Verification items for the finished model (mm, model axes). A direction names the side the tool comes from. Coordinates: 2 decimals unless noted, no trailing zeros. Write each loop counter-clockwise with the first axis right and the second up, starting at its lowest first coordinate (ties: lowest second). Pieces come first, ordered by that corner, then holes. Notation, with made-up numbers: (-33, 81) -> (-14, 81) arc R14 ccw to (-14, 90) -> close; hole circle Ø10 at (-3, 79). An arc over 180 degrees is marked (long way). Answer in a Markdown table with one row per item.
```python
from build123d import *

# Parameters (mm, degrees)
SKETCH_1_R         = 7.5
SKETCH_1_R_2       = 5.25
EXTRUDE_1_DEPTH    = 10
SKETCH_2_R         = 12.5
SKETCH_2_R_2       = 7.5
EXTRUDE_2_DEPTH    = 3
HOLE_WIZARD_M2_1_D = 2.4
CHAMFER_1_SIZE     = 0.5
CHAMFER_2_SIZE     = 0.25


with BuildPart() as part:
    # 草图1 → 凸台-拉伸1 (new body)
    with BuildSketch(Plane(origin=(0, 0, 0), x_dir=(1, 0, 0), z_dir=(0, 1, 0))):
        Circle(SKETCH_1_R)
        Circle(SKETCH_1_R_2, mode=Mode.SUBTRACT)
    extrude(amount=EXTRUDE_1_DEPTH)

    # 草图2 → 凸台-拉伸2 (add)
    with BuildSketch(Plane.XZ):
        Circle(SKETCH_2_R)
        Circle(SKETCH_2_R_2, mode=Mode.SUBTRACT)
    extrude(amount=-EXTRUDE_2_DEPTH)

    # M2 间隙孔1 (through all)
    with Locations(Plane(origin=(-33.948689325, 3, -19.196001998), x_dir=(-0.49220518, 0, 0.870479213), z_dir=(0, 1, 0))):
        with Locations((-10.000000033, 38.999999994), (9.999999967, 38.999999994), (-3.3e-08, 28.999999994)):
            Hole(HOLE_WIZARD_M2_1_D / 2)

    # 倒角1
    chamfer_1_edges = [part.edges().sort_by_distance(p)[0] for p in [
        (-5.25, 10, 0),
    ]]
    chamfer(chamfer_1_edges, length=CHAMFER_1_SIZE)

    # 倒角2
    chamfer_2_edges = [part.edges().sort_by_distance(p)[0] for p in [
        (-9.295438348, 3, -3.877476747),
        (-5.512698019, 3, 9.749367187),
        (4.331405586, 3, -7.660217076),
    ]]
    chamfer(chamfer_2_edges, length=CHAMFER_2_SIZE)


solid = part.part
```
1. Material ranges on probe 1 along Z at (x, y) = (0, 6.5); probe 2 along Y at (x, z) = (-11.25, 2.25), recorded low to high. Write a range as from..to.
Findings below:
| item | result |
|---|---|
| probe 1 | z = -7.5..-5.25, 5.25..7.5 |
| probe 2 | y = 0..3 |
2. Sectioned sample at C-C, the plane y = 7. Record the cut outline in (x, z), and give its area (3 significant figures).
Findings below:
| item | result |
|---|---|
| outline | circle Ø15 at (0, 0); hole circle Ø10.5 at (0, 0) |
| area | 90.1 mm² |
3. Sectioned sample at A-A, the plane x = 0. Record the cut outline in (y, z), and give its area (4 significant figures).
Findings below:
| item | result |
|---|---|
| outline | (0, -12.5) -> (3, -12.5) -> (3, -7.5) -> (10, -7.5) -> (10, -5.75) -> (9.5, -5.25) -> (0, -5.25) -> close; (0, 5.25) -> (9.5, 5.25) -> (10, 5.75) -> (10, 7.5) -> (3, 7.5) -> (3, 12.5) -> (0, 12.5) -> close |
| area | 74.75 mm² |
4. Access from +Z, -Z, +X, -X, +Y, -Y to the whole of each face (thin tool, end or side, straight path). Record for faces 4 (the face through (-9.249, 1.356, -3.853)), 5 (the face through (-7.493, 6.451, -0.33)).
Findings below:
| item | result |
|---|---|
| face 4 | +Y, -Y |
| face 5 | +Y |
5. Go/stop test with flat-tipped pins: pin 1 (2 mm diameter, centred on x = 1.5, y = 1.5, fed in from +Z); pin 2 (3 mm diameter, centred on x = -1.5, y = 6.5, fed in from -Z); pin 3 (5 mm diameter, centred on x = 3.5, y = 7.5, fed in from -Z). Record where each tip stops, or that it passes through.
Findings below:
| item | result |
|---|---|
| pin 1 | stops at z = 12.49 |
| pin 2 | stops at z = -7.5 |
| pin 3 | stops at z = -7.43 |
6. Sectioned sample at B-B, the plane z = 0. Record the cut outline in (x, y).
Findings below:
| item | result |
|---|---|
| outline | (-12.5, 0) -> (-5.25, 0) -> (-5.25, 9.5) -> (-5.75, 10) -> (-7.5, 10) -> (-7.5, 3) -> (-12.5, 3) -> close; (5.25, 0) -> (12.5, 0) -> (12.5, 3) -> (7.5, 3) -> (7.5, 10) -> (5.75, 10) -> (5.25, 9.5) -> close |
7. Release check for a two-part mould opening along X. For faces 1 (the face through (11.923, 1.479, 3.755)), 2 (the face through (8, 3, 0)), 3 (the face through (5.068, 1.356, -9.896)) record: released by +X, released by -X, zero draft, split by the parting line, or undercut.
Findings below:
| item | result |
|---|---|
| face 1 | split by the parting line |
| face 2 | zero draft |
| face 3 | undercut |
8. Sectioned sample at D-D, the plane y = 1. Record the cut outline in (x, z), and give its area (3 significant figures).
Findings below:
| item | result |
|---|---|
| outline | circle Ø25 at (0, 0); hole circle Ø2.4 at (-8.7, -4.92); hole circle Ø2.4 at (-4.92, 8.7); hole circle Ø10.5 at (0, 0); hole circle Ø2.4 at (4.92, -8.7) |
| area | 391 mm² |
